from build123d import *

# Parameters (mm, degrees)
SKETCH_1_R           = 2
EXTRUDE_1_DEPTH      = 2
EXTRUDE_2_DEPTH      = 12.5
EXTRUDE_2_DEPTH_BACK = 2.5
SKETCH_2_R           = 2


with BuildPart() as part:
    # 草图1 → 凸台-拉伸1 (new body)
    with BuildSketch(Plane.XY):
        with BuildLine():
            Line((-6.52657961, 1.983771861), (6.52657961, 1.983771861))
            ThreePointArc((6.52657961, 1.983771861), (14, 0), (6.52657961, -1.983771861))
            Line((6.52657961, -1.983771861), (-6.52657961, -1.983771861))
            ThreePointArc((-6.52657961, -1.983771861), (-14, 0), (-6.52657961, 1.983771861))
        make_face()
        with Locations((-10, 0)):
            Circle(SKETCH_1_R, mode=Mode.SUBTRACT)
        with Locations(Location((10, 0, 0), (0, 0, 180))):
            Circle(SKETCH_1_R, mode=Mode.SUBTRACT)
    extrude_1 = extrude(amount=EXTRUDE_1_DEPTH)

    # 草图2 → 凸台-拉伸2 (add, two sides: drawn at the far end of the back side and taken through both)
    with BuildSketch(Plane.XY.offset(2).offset(-EXTRUDE_2_DEPTH_BACK)):
        with Locations((10, 0)):
            Circle(SKETCH_2_R)
        with Locations((-10, 0)):
            Circle(SKETCH_2_R)
    extrude(amount=EXTRUDE_2_DEPTH + EXTRUDE_2_DEPTH_BACK)

    # 镜向1: 凸台-拉伸1 across plane
    add(extrude_1.mirror(Plane.XY.offset(7)))


solid = part.part
Here's how the part is built. I have some questions about the finished solid (model axes, mm). A direction names the side the tool comes from. Coordinates: 2 decimals unless noted, no trailing zeros. Loops run counter-clockwise (first coordinate to the right, second up) from the corner with the lowest first, then second, coordinate; pieces in that order, holes last. Notation, with made-up numbers: (26.25, 88) -> (69.25, 88) arc R13 cw to (69.25, 111) -> close; hole circle Ø1 at (74, 10). An arc over 180 degrees is marked (long way). Use one line per item in the form item = value. Start each with the question number.
(1) If we section it at C-C (z = 7.75): Please give me the cut outline in (x, y), then the cut area to 3 significant figures.
(2) On a 3-axis mill with a long thin cutter (end or side, diameter ignored), from which of +Z, -Z, +X, -X, +Y, -Y can I reach the whole of each face in a straight line? I mean faces 1 (the face through (-11.6, -1.2, 14.2)), 2 (the face through (0, -1.984, 13)), 3 (the face through (-11.6, -1.2, -0.3)), 4 (the face through (8.4, -1.2, 6.9)). Say none if no direction works.
(3) If we section it at D-D (x = -10): Please give me the cut outline in (y, z), then the cut area to 3 significant figures.
(4) Will these pins go through, and if not, where does the flat tip stop? pin 1 (1.5 mm diameter, centred on y = -1, z = 1, fed in from +X); pin 2 (1 mm diameter, centred on y = -1.5, z = 8.5, fed in from -X); pin 3 (4 mm diameter, centred on y = 2.5, z = 6, fed in from -X); pin 4 (8 mm diameter, centred on x = 9, z = 10.5, fed in from -Y).
(5) If we section it at A-A (x = -6.25): Please give me the cut outline in (y, z).
(6) We'd pull the mould along Z, two halves only. Please class faces 5 (the face through (0, 1.984, 13)), 6 (the face through (0, 0, 12)), 7 (the face through (10, 0, -0.5)), 8 (the face through (0, 0, 2)): pulls with the +Z half, pulls with the -Z half, needs draft (parallel to the pull), parting line crosses it, or undercut.
(7) Please list where these lines run through material, in increasing order: line 1 along Z through (x, y) = (6.25, 1); line 2 along X through (y, z) = (1, 9); line 3 along X through (y, z) = (-3.25, 13.25).
Verdict:
q1.outline = circle Ø4 at (-10, 0); circle Ø4 at (10, 0)
q1.area = 25.1 mm²
q2.face_1 = +Z
q2.face_2 = +Z, -Z, -Y
q2.face_3 = -Z
q2.face_4 = none
q3.outline = (-4, 0) -> (-2, 0) -> (-2, -0.5) -> (2, -0.5) -> (2, 0) -> (4, 0) -> (4, 2) -> (2, 2) -> (2, 12) -> (4, 12) -> (4, 14) -> (2, 14) -> (2, 14.5) -> (-2, 14.5) -> (-2, 14) -> (-4, 14) -> (-4, 12) -> (-2, 12) -> (-2, 2) -> (-4, 2) -> close
q3.area = 76.0 mm²
q4.pin_1 = 13.99
q4.pin_2 = -11.73
q4.pin_3 = -11.94
q4.pin_4 = -4
q5.outline = (-1.98, 0) -> (1.98, 0) -> (1.98, 2) -> (-1.98, 2) -> close; (-1.98, 12) -> (1.98, 12) -> (1.98, 14) -> (-1.98, 14) -> close
q6.face_5 = needs draft
q6.face_6 = undercut
q6.face_7 = pulls with the -Z half
q6.face_8 = undercut
q7.line_1 = 0 to 2, 12 to 14
q7.line_2 = -11.73 to -8.27, 8.27 to 11.73
q7.line_3 = -12.33 to -7.67, 7.67 to 12.33
